Here's how the part is built. I have some questions about the finished solid (model axes, mm). Round coordinates to 2 decimals unless told otherwise and drop trailing zeros. Order: outer loops, then holes, each group sorted by start corner. A loop starts at its lowest first (then second) coordinate and runs counter-clockwise, first axis right, second up. Notation, with made-up numbers: (21, -10) - (39, -10) arc R13 cw to (39, 10) - close; hole circle Ø1 at (4, 62). An arc over 180 degrees is marked (long way). One line per item, written item: value.
from build123d import *

# Parameters (mm, degrees)
F0_W     = 900
F0_H     = 600
F1_DEPTH = 8
F2_W     = 690
F2_H     = 520
F3_DEPTH = 0.3
F4_R     = 3
F5_DEPTH = 2


with BuildPart() as f1:
    # F0 (on Front) → F1 (new body)
    with BuildSketch(Plane.XZ):
        Rectangle(F0_W, F0_H)
    extrude(amount=F1_DEPTH)

    # F2 (on face) → F3 (cut)
    with BuildSketch(Plane.XZ.offset(8)):
        with Locations((-65, 0)):
            Rectangle(F2_W, F2_H)
    extrude(amount=-F3_DEPTH, mode=Mode.SUBTRACT)

    # F4 (on face) → F5 (cut)
    with BuildSketch(Plane.XZ.offset(8)):
        with Locations((392.5, 100)):
            Circle(F4_R)
        with Locations((392.5, 150)):
            Circle(F4_R)
        with Locations((415, -65)):
            Circle(F4_R)
        with Locations((392.5, 50)):
            Circle(F4_R)
        with Locations((355, -50)):
            Circle(F4_R)
        with Locations((415, -50)):
            Circle(F4_R)
        with Locations((415, -175)):
            Circle(F4_R)
        with Locations((415, -205)):
            Circle(F4_R)
        with Locations((415, -235)):
            Circle(F4_R)
        with Locations((415, -265)):
            Circle(F4_R)
        with Locations((355, -265)):
            Circle(F4_R)
        with Locations((355, -65)):
            Circle(F4_R)
        with Locations((355, -175)):
            Circle(F4_R)
        with Locations((355, -205)):
            Circle(F4_R)
        with Locations((355, -235)):
            Circle(F4_R)
        with Locations((392.5, 200)):
            Circle(F4_R)
        with Locations((392.5, 250)):
            Circle(F4_R)
    extrude(amount=-F5_DEPTH, mode=Mode.SUBTRACT)


solid = f1.part
Q1. If we section it at A-A, the plane x = 255.5: Please give me the cut outline in (y, z).
Results list:
outline: (-8, -300) - (0, -300) - (0, 300) - (-8, 300) - (-8, 260) - (-7.7, 260) - (-7.7, -260) - (-8, -260) - close
Q2. If we section it at B-B, the plane z = 79: Please give me the cut outline in (x, y), then the cut area to 3 significant figures.
Results list:
outline: (-450, -8) - (-410, -8) - (-410, -7.7) - (280, -7.7) - (280, -8) - (450, -8) - (450, 0) - (-450, 0) - close
area: 6,990 mm²
Q3. If I drill on line 1 along X through (y, z) = (-7, -175); line 2 along Z through (x, y) = (392.5, -6.9); line 3 along X through (y, z) = (-6.5, -203), over which ranges is the centre line in solid material (lowest first)?
Results list:
line 1: -450 to 352, 358 to 412, 418 to 450
line 2: -300 to 47, 53 to 97, 103 to 147, 153 to 197, 203 to 247, 253 to 300
line 3: -450 to 352.76, 357.24 to 412.76, 417.24 to 450
Q4. Will these pins go through, and if not, where does the flat tip stop? pin 1 (8 mm diameter, centred on x = 355, z = -50, fed in from +Y); pin 2 (1.8 mm diameter, centred on x = 392, z = 201.5, fed in from -Y).
Results list:
pin 1: y = 0
pin 2: y = -6
